from build123d import *

# Parameters (mm, degrees)
SKETCH1_R                           = 14.2875
BOSS_EXTRUDE1_DEPTH                 = 6.35
F_0_257_DIAMETER_HOLE1_D            = 6.5278
F_9_0_2_DIAMETER_HOLE1_D            = 5.08
FILLET2_R                           = 12.7
FILLET1_R                           = 19.05
F_9_0_196_DIAMETER_HOLE1_AT_2_COUNT = 2
F_9_0_196_DIAMETER_HOLE1_AT_2_PITCH = 25.4
F_9_0_196_DIAMETER_HOLE1_AT_3_COUNT = 2
F_9_0_196_DIAMETER_HOLE1_AT_3_PITCH = 76.2
F_9_0_196_DIAMETER_HOLE1_AT_4_COUNT = 2
F_9_0_196_DIAMETER_HOLE1_AT_4_PITCH = 101.6
F_9_0_196_DIAMETER_HOLE2_OUTLINE_R  = 2.4892
F_9_0_196_DIAMETER_HOLE2_DEPTH      = 6.35


# Read off the part's stored shape, not the designer's step: #9 (0.196) Diameter Hole2
with BuildPart() as part:
    # Sketch1 → Boss-Extrude1 (new body)
    with BuildSketch(Plane.YZ):
        with BuildLine():
            Line((0, -50.8), (-201.989896777, -50.8))
            ThreePointArc((-201.989896777, -50.8), (-204.733971085, -38.269563411), (-206.701492618, -25.593970963))
            Line((-206.701492618, -25.593970963), (-265.489896777, -25.593970963))
            Line((-265.489896777, -25.593970963), (-265.489896777, 50.8))
            Line((-265.489896777, 50.8), (-201.989896777, 50.8))
            Line((-201.989896777, 50.8), (0, 50.8))
            ThreePointArc((0, 50.8), (50.8, 0), (0, -50.8))
        make_face()
        with Locations(Location((0, 0, 0), (0, 0, 270))):
            Circle(SKETCH1_R, mode=Mode.SUBTRACT)
        with Locations(Location((-233.739896777, 12.603014519, 0), (0, 0, 270))):
            Circle(SKETCH1_R, mode=Mode.SUBTRACT)
    extrude(amount=BOSS_EXTRUDE1_DEPTH)

    # F (0.257) Diameter Hole1 (through all)
    with Locations(Plane.YZ.offset(6.35)):
        with Locations((0, 0), (-191.833069099, -38.1), (-195.58, 0), (-191.833069099, 38.1)):
            Hole(F_0_257_DIAMETER_HOLE1_D / 2)

    # #9 (0.2) Diameter Hole1 (through all)
    with Locations(Plane.YZ.offset(6.35)):
        with Locations((-259.139896777, 12.603014519), (-208.339896777, 12.603014519)):
            Hole(F_9_0_2_DIAMETER_HOLE1_D / 2)

    # Fillet2
    fillet2_edges = [part.edges().sort_by_distance(p)[0] for p in [
        (3.175, -265.489896777, -25.593970963),
        (3.175, -265.489896777, 50.8),
    ]]
    fillet(fillet2_edges, radius=FILLET2_R)

    # Fillet1
    fillet1_edges = [part.edges().sort_by_distance(p)[0] for p in [
        (3.175, -206.701492618, -25.593970963),
    ]]
    fillet(fillet1_edges, radius=FILLET1_R)

    # Sketch9 → #9 (0.196) Diameter Hole1 (revolve, cut)
    with BuildSketch(Plane(origin=(6.35, -163.889896777, -38.1), x_dir=(0, 0, -1), z_dir=(0, 1, 0))):
        Polygon((0, 0), (0, 6.35), (4.7625, 6.35), (2.4892, 4.0767), (2.4892, 0), align=None)
    f_9_0_196_diameter_hole1 = revolve(axis=Axis((12.7, -163.889896777, -38.1), (-1, 0, 0)), mode=Mode.SUBTRACT)

    # #9 (0.196) Diameter Hole1 at 2: #9 (0.196) Diameter Hole1 ×2
    with Locations(*[(0, i * F_9_0_196_DIAMETER_HOLE1_AT_2_PITCH, 0) for i in range(1, F_9_0_196_DIAMETER_HOLE1_AT_2_COUNT)]):
        add(f_9_0_196_diameter_hole1, mode=Mode.SUBTRACT)

    # #9 (0.196) Diameter Hole1 at 3: #9 (0.196) Diameter Hole1 ×2
    with Locations(*[(0, i * F_9_0_196_DIAMETER_HOLE1_AT_3_PITCH, 0) for i in range(1, F_9_0_196_DIAMETER_HOLE1_AT_3_COUNT)]):
        add(f_9_0_196_diameter_hole1, mode=Mode.SUBTRACT)

    # #9 (0.196) Diameter Hole1 at 4: #9 (0.196) Diameter Hole1 ×2
    with Locations(*[(0, i * F_9_0_196_DIAMETER_HOLE1_AT_4_PITCH, 0) for i in range(1, F_9_0_196_DIAMETER_HOLE1_AT_4_COUNT)]):
        add(f_9_0_196_diameter_hole1, mode=Mode.SUBTRACT)

    # #9 (0.196) Diameter Hole2 outline → #9 (0.196) Diameter Hole2 (cut)
    with BuildSketch(Plane.YZ):
        with Locations((-17.960512242, -17.960512242)):
            Circle(F_9_0_196_DIAMETER_HOLE2_OUTLINE_R)
        with Locations((17.960512242, -17.960512242)):
            Circle(F_9_0_196_DIAMETER_HOLE2_OUTLINE_R)
        with Locations((17.960512242, 17.960512242)):
            Circle(F_9_0_196_DIAMETER_HOLE2_OUTLINE_R)
        with Locations((-17.960512242, 17.960512242)):
            Circle(F_9_0_196_DIAMETER_HOLE2_OUTLINE_R)
    extrude(amount=F_9_0_196_DIAMETER_HOLE2_DEPTH, mode=Mode.SUBTRACT)


solid = part.part
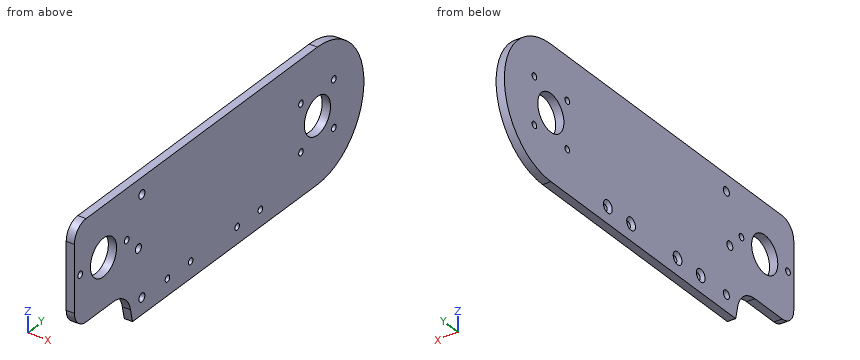
Source: CAD feature listing. Evaluate the final solid. Frame: model axes, mm. Give positions to 0.01 mm unless a question says otherwise; leave off trailing zeros. Return JSON: item names as keys, results as strings. Group by question number.
1) Cut plane A-A, the plane x = 4. Give the number of separate pieces and of enclosed holes in the cut face, plus the area to 3 significant figures.
2) Pin query (flat end, axial travel): P1, Ø1.9, axis at x = 3.5, y = -235, coming from the -Z side; P2, Ø23, axis at y = -233.74, z = 12.6, coming from the +X side; P3, Ø5.5, axis at y = -163.89, z = -38.1, coming from the -X side. Return the tip coordinate at first contact, or that it passes through.
3) Material intervals for line 1 along Y through (x, z) = (1.5, 17); line 2 along Y through (x, z) = (4.25, 9); line 3 along Y through (x, z) = (5.25, 18), sorted ascending. Write a range as [from, to].
Recorded:
{
 "1": {"separate pieces": "1", "enclosed holes": "15", "area": "27,900 mm²"},
 "2": {"P1": "stops at z = -25.59", "P2": "passes through", "P3": "stops at x = 2.01"},
 "3": {"line 1": "y = [-265.49, -247.33], [-220.15, -20.26], [-15.66, 15.66], [20.26, 47.87]", "line 2": "y = [-265.49, -247.57], [-219.91, -11.1], [11.1, 50]", "line 3": "y = [-265.49, -246.97], [-220.51, -20.45], [-15.47, 15.47], [20.45, 47.5]"}
}
